```python
from build123d import *

# Parameters (mm, degrees)
BOSS_EXTRUDE1_DEPTH = 19.05
CUT_EXTRUDE1_START  = -16.51
SKETCH2_R           = 15.875
CUT_EXTRUDE1_DEPTH  = 16.51


with BuildPart() as part:
    # Sketch1 → Boss-Extrude1 (new body)
    with BuildSketch(Plane(origin=(0, 0, 0), x_dir=(1, 0, 0), z_dir=(0, 1, 0))):
        with BuildLine():
            Line((0, -4.7625), (137.850322169, -4.7625))
            ThreePointArc((137.850322169, -4.7625), (161.0950956, -24.394477921), (152.4, 4.7625))
            Line((152.4, 4.7625), (0, 4.7625))
            ThreePointArc((0, 4.7625), (-4.7625, 0), (0, -4.7625))
        make_face()
    extrude(amount=BOSS_EXTRUDE1_DEPTH)

    # Sketch2 → Cut-Extrude1 (cut)
    with BuildSketch(Plane(origin=(0, 19.05, 0), x_dir=(1, 0, 0), z_dir=(0, 1, 0)).offset(CUT_EXTRUDE1_START)):
        with Locations((152.4, -11.1125)):
            Circle(SKETCH2_R)
    extrude(amount=CUT_EXTRUDE1_DEPTH, mode=Mode.SUBTRACT)


solid = part.part
```
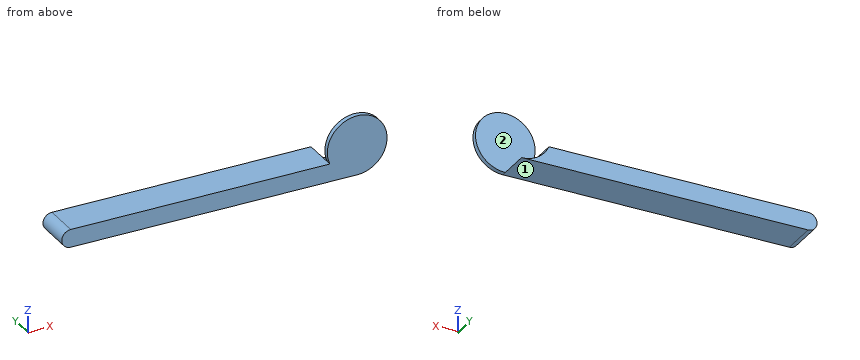
Can you work these out from the model? Positions are in its coordinate system, mm. Face numbers are marked on the shaded views. A direction names the side the tool comes from. Coordinates: 2 decimals unless noted, no trailing zeros. Loops run counter-clockwise (first coordinate to the right, second up) from the corner with the lowest first, then second, coordinate; pieces in that order, holes last. Notation, with made-up numbers: M 19,73.5 L 69,73.5 A5 ccw 69,81.5 Z; hole C 62,30.25 d11. An arc over 180 degrees is marked long. Put each result on its own line as item: value. Start each with the question number.
(1) I need wall thicknesses on probe 1 along Z at (x, y) = (64, 11); probe 2 along Z at (x, y) = (140.5, 1.25); probe 3 along X at (y, z) = (11.75, 2). Which ranges of each line are inside material? Lowest first, please.
(2) Will these pins go through, and if not, where does the flat tip stop? pin 1 Ø1 at (y, z) = (11.5, 1) entering from -X; pin 2 Ø6 at (x, y) = (65, 9.5) entering from +Z.
(3) Which directions (+Z, -Z, +X, -X, +Y, -Y) give clear straight access to the entire face, cutting with the end or side of a thin tool? Please do the marked faces 1 and 2.
(4) Imagine slicing it at C-C on z = 0. List the corners of the cut face in (x, y) for me.
(5) Imagine slicing it at A-A on x = 66. List the corners of the cut face in (y, z) for me, and give its area (3 significant figures).
Worked answers:
1. probe 1: z = -4.76 to 4.76
1. probe 2: z = -4.76 to 21.62
1. probe 3: x = -4.32 to 139.4
2. pin 1: stops at x = -4.74
2. pin 2: stops at z = 4.76
3. face 1: -Z, +X, -X, +Y, -Y
3. face 2: +Z, +X, +Y
4. outline: M -4.76,0 L 163.74,0 L 163.74,2.54 L 141.06,2.54 L 141.06,19.05 L -4.76,19.05 Z
5. outline: M 0,-4.76 L 19.05,-4.76 L 19.05,4.76 L 0,4.76 Z
5. area: 181 mm2
